Source: CAD feature listing. Evaluate the final solid. Frame: model axes, mm. Face numbers are marked on the shaded views. Coordinates: 2 decimals unless noted, no trailing zeros. One line per item, written item: value. Start each with the question number.
Item 1: Pin query (flat end, axial travel): P1, Ø6.5, axis at x = 6.761, z = -16.682, coming from the +Y side; P2, Ø4.5, axis at x = 18, z = 0, coming from the -Y side; P3, Ø2, axis at x = 20, y = 2.5, coming from the -Z side. Return the tip coordinate at first contact, or that it passes through.
Item 2: Ray query, L1, parallel to Z at x = 0, y = 2; L2, parallel to Z at x = -7, y = 3.5; L3, parallel to X at y = 6.5, z = 11.5. Return the intervals inside material, ascending. Write a range as from..to.
Item 3: Cut plane A-A, the plane x = 0. State how many separate pieces and enclosed holes the cut face has, then the cut area to 3 significant figures.
Item 4: Mould query, pull axis Z, two halves, no side actions, for the marked faces 1, 2 and 3. Classes: released by +Z, released by -Z, zero draft, split by the parting line, or undercut.
Autodesk Inventor part; units mm, degrees
ref_plane "Work Plane2" through (0, 0, 0) normal (0.3827, 0, 0.9239) x (0, 1, 0)
ref_plane "YZ Plane" through (0, 0, 0) normal (1, 0, 0) x (0, 1, 0)
ref_plane "XZ Plane" through (0, 0, 0) normal (0, 1, 0) x (-1, 0, 0)
sketch "Sketch1" plane through (0, 0, 0) normal (0, 1, 0) x (-1, 0, 0)
  circle A0 centre (0, 0) radius 6
  circle A1 centre (0, 0) radius 25
  circle A2 centre (0, -18) radius 2
  circle A3 centre (12.7279, -12.7279) radius 2
  circle A4 centre (18, 0) radius 2
  circle A5 centre (12.7279, 12.7279) radius 2
  circle A6 centre (0, 18) radius 2
  circle A7 centre (-12.7279, 12.7279) radius 2
  circle A8 centre (-18, 0) radius 2
  circle A9 centre (-12.7279, -12.7279) radius 2
  circle A10 centre (16.682, -6.761) radius 2
  circle A11 centre (6.761, 16.682) radius 2
  circle A12 centre (-16.682, 6.761) radius 2
  circle A13 centre (-6.761, -16.682) radius 2
  dimension "d0" = 50
  dimension "d1" = 12
  dimension "d4" = 4
  dimension "d5" = 18
  dimension "d8" = 360
  dimension "d18" = 4
  dimension "d21" = 13.7766
  dimension "d22" = 6.8883
  dimension "d23" = 18
  dimension "d26" = 360
extrude "Extrusion1" add sketch "Sketch1" along normal blind 8
ref_plane "Work Plane2" through (0, 0, 0) normal (0.3827, 0, 0.9239) x (0, 1, 0)
sketch "Sketch2" plane through (0, 0, 0) normal (0.3827, 0, 0.9239) x (0, 1, 0)
  circle A0 centre (4, 0) radius 1.5
  line L0 (8, -25) -> (8, 25)
  line L1 (0, -25) -> (0, 25)
  point P0 (0, 0)
  dimension "d11" = 3
  dimension "d12" = 8
  dimension "d13" = 4
extrude "Extrusion2" cut sketch "Sketch2" against normal up to surface
thread "Thread1"
chamfer "Chamfer1" distance 1.5 angle 45 4 edges at (18.682, 8, 6.761) (-4.761, 8, 16.682) (-14.682, 8, -6.761) (8.761, 8, -16.682)
thread "Thread2"
thread "Thread3"
thread "Thread4"
thread "Thread5"
thread "Thread6"
thread "Thread7"
thread "Thread8"
thread "Thread9"
chamfer "Chamfer2" distance 0.5 angle 45 25 edges at (25, 8, 0) (6, 8, 0) (25, 0, 0) (6, 0, 0) (14.7279, 8, -12.7279) (20, 8, 0) (14.7279, 8, 12.7279) (2, 8, 18) (-10.7279, 8, 12.7279) (-16, 8, 0) (-10.7279, 8, -12.7279) (2, 8, -18) (-10.0215, 2.5836, -22.9035) (2, 0, -18) (8.761, 0, -16.682) (14.7279, 0, -12.7279) (20, 0, 0) (18.682, 0, 6.761) (14.7279, 0, 12.7279) (2, 0, 18) (-4.761, 0, 16.682) (-10.7279, 0, 12.7279) (-16, 0, 0) (-14.682, 0, -6.761) (-10.7279, 0, -12.7279)
pattern_circular "Circular Pattern1" count 2 over 90 about axis through (0, -10, 0) along (0, 1, 0) of "Extrusion2"
equation "\"d22\" = 0.5 * d21"
equation "\"d13\" = 0.5 * d12"
properties part number "endeffector mount part"
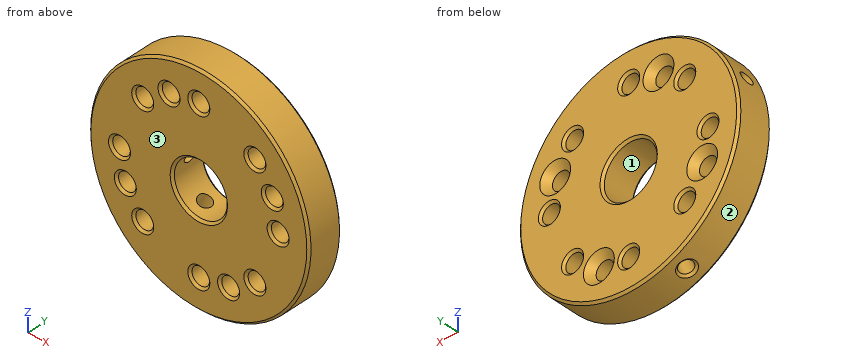
From the geometry:
1. P1: stops at y = 7.75
1. P2: stops at y = 0.25
1. P3: stops at z = -16.25
2. L1: z = -25..-20, -16..-6, 6..16, 20..25
2. L2: z = -24..-20.6, -13.2..1.37, 4.43..14.7, 18.67..24
2. L3: x = -22.2..-14.31, -11.15..11.15, 14.31..22.2
3. separate pieces: 4
3. enclosed holes: 0
3. area: 238 mm²
4. face 1: undercut
4. face 2: split by the parting line
4. face 3: zero draft
